The listing builds one solid part. Answer for the finished solid, in the listing's coordinates (mm). A direction names the side the tool comes from. Round coordinates to 2 decimals unless told otherwise and drop trailing zeros. Order: outer loops, then holes, each group sorted by start corner. A loop starts at its lowest first (then second) coordinate and runs counter-clockwise, first axis right, second up. Notation, with made-up numbers: (69, -24) - (104, -24) arc R23 ccw to (104, -7) - close; hole circle Ø6 at (46, 86.25). An arc over 180 degrees is marked (long way). Use CSV: the item, a comma, the result in double quotes. Start each with the question number.
Item 1: For faces 4 (the cylindrical face through (4.74, -3.39, 0.49)), 5 (the cylindrical face through (-5.895, -6.395, 0.493)), determine the directions among +Z, -Z, +X, -X, +Y, -Y from which every point of the face is accessible in a straight line to the end or side of a thin tool.
Item 2: Find section B-B, the plane z = 0.6. Give the vertices of the cut face in (x, y) (3 decimals), plus the area to 3 significant figures.
Item 3: Straight lines are drawn through the part: line 1 along Y through (x, z) = (-3.75, 0.1); line 2 along Y through (x, z) = (-3.5, 0.45); line 3 along X through (y, z) = (0, 0.2). For each, find the intervals that lie inside material, in ascending order. Write a range as [from, to].
Item 4: Determine the mould class of faces 1 (the cylindrical face through (-2.12, -4.4, 0.49)), 2 (the flat face through (0, 7, 1)), 3 (the cylindrical face through (0.271, 9.246, 0.493)) for opening direction X: +X half, -X half, draft (parallel to the pull), parting line (faces both ways), or undercut.
Item 5: Find section D-D, the plane x = 0. Give the vertices of the cut face in (y, z).
Item 6: Find section A-A, the plane y = 0. Give the vertices of the cut face in (x, z).
Item 7: A flat-ended cylindrical pin translates along its axis: P1, Ø0.9, axis at x = -3.62, y = -4.9, coming from the +Z side. Find the tip coordinate at first contact, or state that the pin passes through.
Item 8: Find section C-C, the plane y = 3. Give the vertices of the cut face in (x, z).
```python
from build123d import *

# Parameters (mm, degrees)
F0_R     = 0.75
F1_DEPTH = 1


with BuildPart() as f1:
    # F0 (on Top) → F1 (new body)
    with BuildSketch(Plane.XY):
        with BuildLine():
            ThreePointArc((-5.196152, -3), (0, 6), (5.196152, -3))
            ThreePointArc((5.196152, -3), (4.736217, -3.390004), (4.133261, -3.399364))
            ThreePointArc((4.133261, -3.399364), (2.132517, -4.362657), (3.062402, -6.379145))
            ThreePointArc((3.062402, -6.379145), (5.857871, -6.408447), (8.010735, -4.625))
            ThreePointArc((8.010735, -4.625), (0, 9.25), (-8.010735, -4.625))
            ThreePointArc((-8.010735, -4.625), (-5.857871, -6.408447), (-3.062402, -6.379145))
            ThreePointArc((-3.062402, -6.379145), (-2.132517, -4.362657), (-4.133261, -3.399364))
            ThreePointArc((-4.133261, -3.399364), (-4.736217, -3.390004), (-5.196152, -3))
        make_face()
        with Locations((-3.622614, -4.898161)):
            Circle(F0_R, mode=Mode.SUBTRACT)
        with Locations((3.622614, -4.898161)):
            Circle(F0_R, mode=Mode.SUBTRACT)
    extrude(amount=F1_DEPTH)


solid = f1.part
```
Worked out:
1,face 4,"+Z, -Z"
1,face 5,"+Z, -Z, -Y"
2,outline,"(-8.011, -4.625) arc R4.064 ccw to (-3.062, -6.379) arc R1.583 ccw to (-4.133, -3.399) arc R0.894 cw to (-5.196, -3) arc R6 cw (long way) to (5.196, -3) arc R0.894 cw to (4.133, -3.399) arc R1.583 ccw to (3.062, -6.379) arc R4.064 ccw to (8.011, -4.625) arc R9.25 ccw (long way) to start; hole circle Ø1.5 at (-3.623, -4.898); hole circle Ø1.5 at (3.623, -4.898)"
2,area,"130 mm²"
3,line 1,"y = [-6.57, -5.64], [-4.16, -3.32], [4.68, 8.46]"
3,line 2,"y = [-6.52, -5.64], [-4.16, -3.32], [4.87, 8.56]"
3,line 3,"x = [-9.25, -6], [6, 9.25]"
4,face 1,"undercut"
4,face 2,"draft"
4,face 3,"parting line"
5,outline,"(6, 0) - (9.25, 0) - (9.25, 1) - (6, 1) - close"
6,outline,"(-9.25, 0) - (-6, 0) - (-6, 1) - (-9.25, 1) - close; (6, 0) - (9.25, 0) - (9.25, 1) - (6, 1) - close"
7,P1,"passes through"
8,outline,"(-8.75, 0) - (-5.2, 0) - (-5.2, 1) - (-8.75, 1) - close; (5.2, 0) - (8.75, 0) - (8.75, 1) - (5.2, 1) - close"
